```python
from build123d import *

# Parameters (mm, degrees)
EXTRUS_O_PRINCIPAL_DEPTH    = 250
ESCALA_SCALE                = 1.5
ALIVIO_START                = -75
ALIVIO_SUP_INF_DEPTH        = 225
AL_VIO_CENTRAL_DEPTH        = 344.797069556
AL_VIO_CENTRAL_DEPTH_BACK   = 344.797069556
FUROS_DIR_D                 = 8.5
FUROS_DIR_DEPTH             = 27.5
FUROS_DIR_CSINK_D           = 10.05
FUROS_DIR_CSINK_ANGLE       = 90
FUROS_DIR_TIP               = 2.553657631
FUROS_ESQ_D                 = 8.5
FUROS_ESQ_DEPTH             = 27.5
FUROS_ESQ_CSINK_D           = 10.05
FUROS_ESQ_CSINK_ANGLE       = 90
FUROS_ESQ_TIP               = 2.553657631
ESBO_O7_3_R                 = 25
FURO_EIXO_DEPTH             = 395.584089109
ESBO_O7_R                   = 36
REBAIXO_ROLAMENTO_ESQ_DEPTH = 69
REBAIXO_START               = -306
ESBO_O7_4_R                 = 36
ESBO_O7_4_R_2               = 25
REBAIXO_ROLAMENTO_DIR_DEPTH = 69


with BuildPart() as part:
    # Esboço1 → EXTRUSÃO PRINCIPAL (new body)
    with BuildSketch(Plane.XY):
        with BuildLine():
            Line((65, 0), (64.021024633, -14))
            Line((64.021024633, -14), (56.886629039, -33.601590794))
            Line((56.886629039, -33.601590794), (-36.113370961, -50))
            Line((-36.113370961, -50), (-51.485110725, -44.405144277))
            Line((-51.485110725, -44.405144277), (-62, -31.873987208))
            Line((-62, -31.873987208), (-62, 9.746573698))
            Line((-62, 9.746573698), (-54, 26.190795203))
            Line((-54, 26.190795203), (-36.113370961, 29.996175937))
            Line((-36.113370961, 29.996175937), (27, 20))
            Line((27, 20), (32.013345877, 9.746573698))
            ThreePointArc((32.013345877, 9.746573698), (40.293006212, 1.034435734), (52.07121536, -1.358870022))
            Line((52.07121536, -1.358870022), (65, 0))
        make_face()
    extrude(amount=EXTRUS_O_PRINCIPAL_DEPTH)


with BuildPart() as part_1:
    # ESCALA: scaled about (-7.179170438, -10.680236315, 125)
    add(part.part.scale(ESCALA_SCALE).moved(Location((3.589585219, 5.340118158, -62.5))))

    # Esboço4 → ALIVIO SUP./INF. (cut)
    with BuildSketch(Plane(origin=(0, 0, -62.5), x_dir=(-1, 0, 0), z_dir=(0, 0, -1)).offset(ALIVIO_START)):
        Polygon((89.410414781, 12.959978704), (89.410414781, 19.959978704), (77.410414781, 44.626310962), (50.580471222, 50.334382062), (-44.089585219, 35.340118158), align=None)
        Polygon((73.638080869, -61.267598258), (89.410414781, -42.470862654), (-88.919528778, -45.062268034), (50.580471222, -69.659881842), align=None)
    extrude(amount=-ALIVIO_SUP_INF_DEPTH, mode=Mode.SUBTRACT)

    # Esboço6 → ALÍVIO CENTRAL (cut, two sides: drawn at the far end of the back side and taken through both)
    with BuildSketch(Plane(origin=(-4.557313786, 27.184879328, 0), x_dir=(0.9862375757372075, 0.16533434066761868, 0), z_dir=(-0.16533434066761868, 0.9862375757372075, 0)).offset(-AL_VIO_CENTRAL_DEPTH_BACK)):
        with BuildLine():
            Line((-36.037181185, -37.5), (-0.674259224, -37.5))
            ThreePointArc((-0.674259224, -37.5), (17.003410306, -44.82233047), (24.325740776, -62.5))
            Line((24.325740776, -62.5), (24.325740776, -187.5))
            ThreePointArc((24.325740776, -187.5), (17.003410306, -205.17766953), (-0.674259224, -212.5))
            Line((-0.674259224, -212.5), (-36.037181185, -212.5))
            ThreePointArc((-36.037181185, -212.5), (-53.714850715, -205.17766953), (-61.037181185, -187.5))
            Line((-61.037181185, -187.5), (-61.037181185, -62.5))
            ThreePointArc((-61.037181185, -62.5), (-53.714850715, -44.82233047), (-36.037181185, -37.5))
        make_face()
    extrude(amount=AL_VIO_CENTRAL_DEPTH + AL_VIO_CENTRAL_DEPTH_BACK, mode=Mode.SUBTRACT)

    # FUROS DIR.
    with Locations(Plane.XY.offset(312.5)):
        with Locations((53.280280787, -11.103047714), (-39.437052477, 22.643301795), (-51.681610143, -9.103047714), (-42.225201538, -41.215810622), (48.741417313, -32.456721475)):
            CounterSinkHole(FUROS_DIR_D / 2, FUROS_DIR_CSINK_D / 2, depth=FUROS_DIR_DEPTH, counter_sink_angle=FUROS_DIR_CSINK_ANGLE)
            with Locations((0, 0, -(FUROS_DIR_DEPTH + FUROS_DIR_TIP / 2))):  # 118° drill point
                Cone(0, FUROS_DIR_D / 2, FUROS_DIR_TIP, mode=Mode.SUBTRACT)

    # FUROS ESQ.
    with Locations(Plane(origin=(0, 0, -62.5), x_dir=(-1, 0, 0), z_dir=(0, 0, -1))):
        with Locations((39.437052477, 22.643301795), (51.681610143, -9.103047714), (42.225201538, -41.215810622), (-48.741417313, -32.456721475), (-53.280280787, -11.103047714)):
            CounterSinkHole(FUROS_ESQ_D / 2, FUROS_ESQ_CSINK_D / 2, depth=FUROS_ESQ_DEPTH, counter_sink_angle=FUROS_ESQ_CSINK_ANGLE)
            with Locations((0, 0, -(FUROS_ESQ_DEPTH + FUROS_ESQ_TIP / 2))):  # 118° drill point
                Cone(0, FUROS_ESQ_D / 2, FUROS_ESQ_TIP, mode=Mode.SUBTRACT)

    # Esboço7<3> → FURO EIXO (cut, through all)
    with BuildSketch(Plane.XY.offset(312.5)):
        with Locations((0.809103247, -11.098343232)):
            Circle(ESBO_O7_3_R)
    extrude(amount=-FURO_EIXO_DEPTH, mode=Mode.SUBTRACT)

    # Esboço7 → REBAIXO ROLAMENTO ESQ. (cut)
    with BuildSketch(Plane.XY.offset(312.5)):
        with Locations((0.809103247, -11.098343232)):
            Circle(ESBO_O7_R)
    extrude(amount=-REBAIXO_ROLAMENTO_ESQ_DEPTH, mode=Mode.SUBTRACT)

    # Esboço7<4> → REBAIXO ROLAMENTO DIR. (cut)
    with BuildSketch(Plane.XY.offset(312.5).offset(REBAIXO_START)):
        with Locations((0.809103247, -11.098343232)):
            Circle(ESBO_O7_4_R)
        with Locations(Location((0.809103247, -11.098343232, 0), (0, 0, 280.347956823))):
            Circle(ESBO_O7_4_R_2, mode=Mode.SUBTRACT)
    extrude(amount=-REBAIXO_ROLAMENTO_DIR_DEPTH, mode=Mode.SUBTRACT)


solid = part_1.part
```
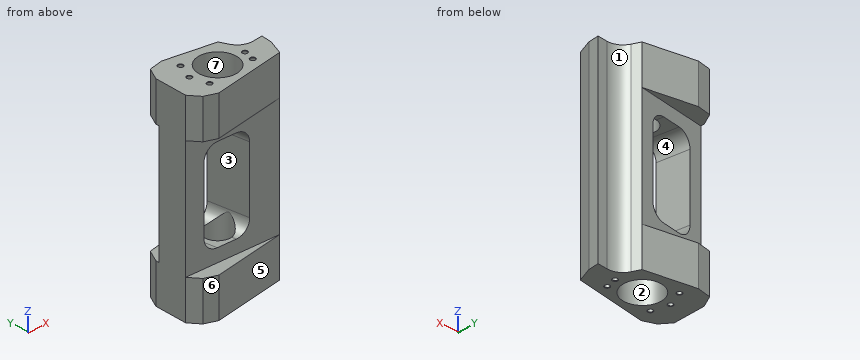
Model file for the job. Use its own axes, mm. Face numbers are marked on the shaded views. A direction names the side the tool comes from. Give positions to 0.01 mm unless a question says otherwise; leave off trailing zeros. Loops run counter-clockwise (first coordinate to the right, second up) from the corner with the lowest first, then second, coordinate; pieces in that order, holes last. Notation, with made-up numbers: (1.5, -39) -> (51.5, -39) arc R23 ccw to (51.5, -22) -> close; hole circle Ø7 at (-34, 17.25). An arc over 180 degrees is marked (long way). Write each question's results on one line, items separated by ' | '.
(1) Probe line 1 along Z through (x, y) = (-49, -56); line 2 along X through (y, z) = (-38.5, -4.5); line 3 along X through (y, z) = (-21.5, 118). List the from-to ranges inside material, lowest first.
Geometry results:
line 1: z = -62.5 to 12.5, 237.5 to 312.5 | line 2: x = -89.41 to -22.54, 24.16 to 91.31 | line 3: x = -89.41 to -58.28, 28.27 to 97.5
(2) Cut at C-C on x = -15.5. Give the number of separate pieces and of enclosed holes in the cut face, and give its area (3 significant figures).
Geometry results:
separate pieces: 4 | enclosed holes: 0 | area: 8,480 mm²
(3) Cut at D-D on z = 234. List the corners of the cut face in (x, y).
Geometry results:
outline: (-89.41, -42.47) -> (88.92, -45.06) -> (99.62, -15.66) -> (101.09, 5.34) -> (81.7, 3.3) arc R30 cw to (51.61, 19.96) -> (44.09, 35.34) -> (-89.41, 12.96) -> close; hole circle Ø50 at (0.81, -11.1)
(4) Flat gauge pins, fed straight in: pin 1 Ø8 at (y, z) = (-37, 241.5) entering from +X; pin 2 Ø7.5 at (x, y) = (53.28, -11.1) entering from -Z; pin 3 Ø7.5 at (x, y) = (48.74, -32.46) entering from +Z; pin 4 Ø21.5 at (x, y) = (-0.5, -3.5) entering from -Z. Where does each tip first touch, or does it go through?
Geometry results:
pin 1: stops at x = 93.31 | pin 2: stops at z = -34.7 | pin 3: stops at z = 284.7 | pin 4: passes through
(5) Tool access for the marked faces 1, 2, 3 and 4: list every direction of +Z, -Z, +X, -X, +Y, -Y with a clear straight run to the whole face (end or side of a thin tool).
Geometry results:
face 1: +Z, -Z, +Y | face 2: -Z | face 3: -Y | face 4: +Y
(6) Cut at A-A on z = 156. List the corners of the cut face in (x, y).
Geometry results:
outline: (-89.41, -42.47) -> (-54.68, -42.98) -> (-64.75, 17.09) -> (-89.41, 12.96) -> close; (19.43, 31.21) -> (32.08, -44.24) -> (88.92, -45.06) -> (99.62, -15.66) -> (101.09, 5.34) -> (81.7, 3.3) arc R30 cw to (51.61, 19.96) -> (44.09, 35.34) -> close
(7) Cut at B-B on z = -39.5. List the corners of the cut face in (x, y).
Geometry results:
outline: (-89.41, -42.47) -> (-73.64, -61.27) -> (-50.58, -69.66) -> (88.92, -45.06) -> (99.62, -15.66) -> (101.09, 5.34) -> (81.7, 3.3) arc R30 cw to (51.61, 19.96) -> (44.09, 35.34) -> (-50.58, 50.33) -> (-77.41, 44.63) -> (-89.41, 19.96) -> close; hole circle Ø8.5 at (-51.68, -9.1); hole circle Ø8.5 at (-42.23, -41.22); hole circle Ø8.5 at (-39.44, 22.64); hole circle Ø72 at (0.81, -11.1); hole circle Ø8.5 at (48.74, -32.46); hole circle Ø8.5 at (53.28, -11.1)
(8) Pull direction X, two halves, no side cores. Call the marked faces 5, 6 and 7: released by +X, released by -X, zero draft, split by the parting line, or undercut.
Geometry results:
face 5: released by +X | face 6: released by -X | face 7: undercut
